```python
from build123d import *

# Parameters (mm, degrees)
F0_R     = 2.335
F1_DEPTH = 20.32
F2_R     = 5.08
F2_R_2   = 2.335
F3_DEPTH = 2.54
F4_R     = 0.889
F5_DEPTH = 12.7


with BuildPart() as f1:
    # F0 (on Top) → F1 (new body)
    with BuildSketch(Plane.XY):
        Circle(F0_R)
    extrude(amount=F1_DEPTH)

    # F2 (on face) → F3 (join)
    with BuildSketch(Plane(origin=(0, 0, 0), x_dir=(1, 0, 0), z_dir=(0, 0, -1))):
        Circle(F2_R)
        Circle(F2_R_2, mode=Mode.SUBTRACT)
        Circle(F2_R_2)
    extrude(amount=F3_DEPTH)

    # F4 (on Front) → F5 (cut, symmetric)
    with BuildSketch(Plane.XZ):
        with Locations((0, 18.669)):
            Circle(F4_R)
    extrude(amount=F5_DEPTH, both=True, mode=Mode.SUBTRACT)


solid = f1.part
```
Check sheet for the modelled part. Datum: model origin and axes. Units: mm. A direction names the side the tool comes from. Round coordinates to 2 decimals unless told otherwise and drop trailing zeros. Write each loop counter-clockwise with the first axis right and the second up, starting at its lowest first coordinate (ties: lowest second). Pieces come first, ordered by that corner, then holes. Notation, with made-up numbers: M 54.25,76 L 79.25,76 A35 cw 79.25,110 Z; hole C 12,60 d9. An arc over 180 degrees is marked long. Write item = value, one per line. Start each with the question number.
1. Section check C-C, the plane z = 18.25. Record the cut outline in (x, y) (3 decimals).
2. Release check for a two-part mould opening along Z. For faces 3 (the flat face through (2.2, -1.2, 0)), 4 (the cylindrical face through (-0.661, -5.037, -1.252)), 5 (the cylindrical face through (-0.19, -0.03, 17.8)) record: pulls with the +Z half, pulls with the -Z half, needs draft (parallel to the pull), parting line crosses it, or undercut.
3. Gauge pin test, flat ends, axial feed: pin 1 (3 mm diameter, centred on x = -2, z = 15, fed in from +Y); pin 2 (3 mm diameter, centred on x = 1, z = 8.5, fed in from -Y) (3 decimals); pin 3 (1.5 mm diameter, centred on y = -2.5, z = 3, fed in from +X). Record the tip position at first contact, or that the pin passes through.
4. Scan lines: line 1 (Z direction, x = 0, y = 0.6); line 2 (Z direction, x = 2.5, y = -0.5); line 3 (Z direction, x = -0.25, y = 1). Record each from-to range of solid material in increasing order. Write a range as [from, to].
5. Section check A-A, the plane x = 0. Record the cut outline in (y, z) (3 decimals).
6. Section check B-B, the plane y = -0.5. Record the cut outline in (x, z), then the cut area to 3 significant figures.
7. Tool access check on faces 1 (the flat face through (0, 0, -2.54)), 2 (the cylindrical face through (2.227, 0.701, 10.018)). Record the directions out of +Z, -Z, +X, -X, +Y, -Y that give a thin tool (end or side, any length) a straight path to the whole face; none if there is none.
8. Section check D-D, the plane y = 1. Record the cut outline in (x, z), then the cut area to 3 significant figures.
Results found:
q1.outline = M -0.784,-2.199 L -0.784,2.199 A2.335 ccw Z; M 0.784,-2.199 A2.335 ccw 0.784,2.199 Z
q2.face_3 = pulls with the +Z half
q2.face_4 = needs draft
q2.face_5 = undercut
q3.pin_1 = 2.28
q3.pin_2 = -2.335
q3.pin_3 = 1.55
q4.line_1 = [-2.54, 17.78], [19.56, 20.32]
q4.line_2 = [-2.54, 0]
q4.line_3 = [-2.54, 17.82], [19.52, 20.32]
q5.outline = M -5.08,-2.54 L 5.08,-2.54 L 5.08,0 L 2.335,0 L 2.335,17.78 L -2.335,17.78 L -2.335,0 L -5.08,0 Z; M -2.335,19.558 L 2.335,19.558 L 2.335,20.32 L -2.335,20.32 Z
q6.outline = M -5.06,-2.54 L 5.06,-2.54 L 5.06,0 L 2.28,0 L 2.28,20.32 L -2.28,20.32 L -2.28,0 L -5.06,0 Z; hole C 0,18.67 d1.78
q6.area = 116 mm^2
q7.face_1 = -Z, +X, -X, +Y, -Y
q7.face_2 = +Z
q8.outline = M -4.98,-2.54 L 4.98,-2.54 L 4.98,0 L 2.11,0 L 2.11,20.32 L -2.11,20.32 L -2.11,0 L -4.98,0 Z; hole C 0,18.67 d1.78
q8.area = 109 mm^2
